Could you check a few things on this model? Use its own coordinates, in mm. Coordinates: 2 decimals unless noted, no trailing zeros. Order: outer loops, then holes, each group sorted by start corner. A loop starts at its lowest first (then second) coordinate and runs counter-clockwise, first axis right, second up. Notation, with made-up numbers: (77, 14.5) - (124, 14.5) arc R32 cw to (124, 40.5) - close; hole circle Ø5 at (17.5, -24). An arc over 180 degrees is marked (long way). Answer as a JSON object with one key per item and string values. Group by question number.
(1) Imagine slicing it at A-A, the plane y = 8.75. Write out the boundary of the cut face in (x, z), and give its area (3 significant figures).
(2) Will these pins go through, and if not, where does the flat tip stop? P1, Ø5, axis at x = -24.5, y = 9.5, coming from the -Z side; P2, Ø1, axis at x = -3, y = 16.5, coming from the +Z side; P3, Ø1.5, axis at y = 5.5, z = 15, coming from the -X side.
(3) Please list where these lines run through material, in increasing order: probe 1 along X at (y, z) = (3.25, 0); probe 2 along X at (y, z) = (12, -10).
from build123d import *

# Parameters (mm, degrees)
SKETCH1_R           = 35
BOSS_EXTRUDE1_DEPTH = 25
CHAMFER1_SIZE       = 2
FILLET2_R           = 1


with BuildPart() as part:
    # Sketch1 → Boss-Extrude1 (new body)
    with BuildSketch(Plane(origin=(0, 0, 0), x_dir=(1, 0, 0), z_dir=(0, 1, 0))):
        with Locations(Location((0, 0, 0), (0, 0, 270))):
            Circle(SKETCH1_R)
    extrude(amount=BOSS_EXTRUDE1_DEPTH)

    # Chamfer1
    chamfer1_edges = [part.edges().sort_by_distance(p)[0] for p in [
        (0, 0, -35),
        (0, 25, -35),
    ]]
    chamfer(chamfer1_edges, length=CHAMFER1_SIZE)

    # Fillet2
    fillet2_edges = [part.edges().sort_by_distance(p)[0] for p in [
        (0, 23, -35),
        (0, 2, -35),
        (0, 0, -33),
        (0, 25, -33),
    ]]
    fillet(fillet2_edges, radius=FILLET2_R)


solid = part.part
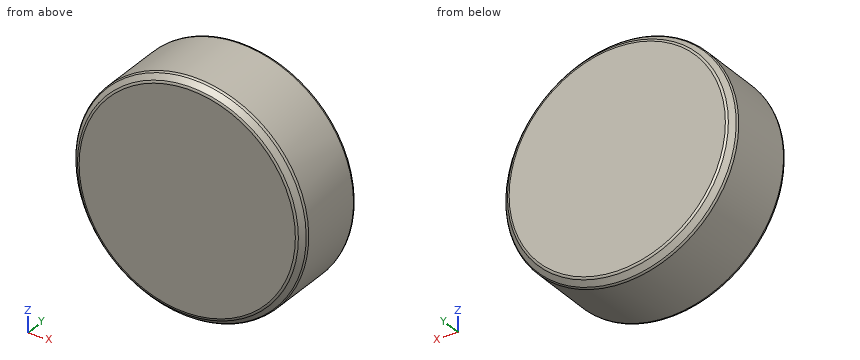
Result set:
{
 "1": {"outline": "circle Ø70 at (0, 0)", "area": "3,850 mm^2"},
 "2": {"P1": "stops at z = -27.22", "P2": "stops at z = 34.91", "P3": "stops at x = -31.97"},
 "3": {"probe 1": "x = -35 to 35", "probe 2": "x = -33.54 to 33.54"}
}
